Here's how the part is built. I have some questions about the finished solid (model axes, mm). Give positions to 0.01 mm unless a question says otherwise; leave off trailing zeros. Loops run counter-clockwise (first coordinate to the right, second up) from the corner with the lowest first, then second, coordinate; pieces in that order, holes last. Notation, with made-up numbers: (-30, -34.75) - (3, -34.75) arc R31 ccw to (3, -4.75) - close; hole circle Ø3 at (-6.75, 86.25). An arc over 180 degrees is marked (long way). Use one line per item in the form item = value.
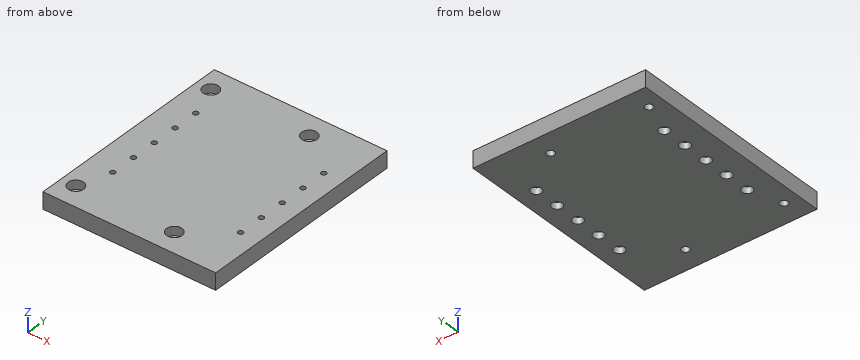
from build123d import *

# Parameters (mm, degrees)
F0_W     = 135
F0_H     = 165
F0_R     = 6
F0_R_2   = 2
F0_R_3   = 3
F1_DEPTH = 13
F2_R     = 6
F3_DEPTH = 7
F4_R     = 4
F5_DEPTH = 5


with BuildPart() as f1:
    # F0 (on Top) → F1 (new body)
    with BuildSketch(Plane.XY):
        with Locations((17.5, 0)):
            Rectangle(F0_W, F0_H)
        with Locations((-38.5, -65)):
            Circle(F0_R, mode=Mode.SUBTRACT)
        with Locations((-30, -40)):
            Circle(F0_R_2, mode=Mode.SUBTRACT)
        with Locations((-30, -20)):
            Circle(F0_R_2, mode=Mode.SUBTRACT)
        with Locations((38.5, -65)):
            Circle(F0_R, mode=Mode.SUBTRACT)
        with Locations((70, -40)):
            Circle(F0_R_2, mode=Mode.SUBTRACT)
        with Locations((70, -20)):
            Circle(F0_R_2, mode=Mode.SUBTRACT)
        with Locations((-30, 0)):
            Circle(F0_R_2, mode=Mode.SUBTRACT)
        with Locations((-30, 20)):
            Circle(F0_R_2, mode=Mode.SUBTRACT)
        with Locations((-30, 40)):
            Circle(F0_R_2, mode=Mode.SUBTRACT)
        with Locations((-38.5, 65)):
            Circle(F0_R, mode=Mode.SUBTRACT)
        with Locations((70, 0)):
            Circle(F0_R_2, mode=Mode.SUBTRACT)
        with Locations((70, 20)):
            Circle(F0_R_2, mode=Mode.SUBTRACT)
        with Locations((70, 40)):
            Circle(F0_R_2, mode=Mode.SUBTRACT)
        with Locations((38.5, 65)):
            Circle(F0_R, mode=Mode.SUBTRACT)
        with Locations((-38.5, 65)):
            Circle(F0_R)
        with Locations((-38.5, 65)):
            Circle(F0_R_3, mode=Mode.SUBTRACT)
        with Locations((38.5, 65)):
            Circle(F0_R)
        with Locations((38.5, 65)):
            Circle(F0_R_3, mode=Mode.SUBTRACT)
        with Locations((38.5, -65)):
            Circle(F0_R)
        with Locations((38.5, -65)):
            Circle(F0_R_3, mode=Mode.SUBTRACT)
        with Locations((-38.5, -65)):
            Circle(F0_R)
        with Locations((-38.5, -65)):
            Circle(F0_R_3, mode=Mode.SUBTRACT)
    extrude(amount=-F1_DEPTH)

    # F0 (on Top) + F2 (on face) → F3 (cut)
    with BuildSketch(Plane.XY):
        with Locations((-38.5, 65)):
            Circle(F0_R)
        with Locations((-38.5, 65)):
            Circle(F0_R_3, mode=Mode.SUBTRACT)
        with Locations((-38.5, 65)):
            Circle(F0_R_3)
        with Locations((38.5, 65)):
            Circle(F0_R)
        with Locations((38.5, 65)):
            Circle(F0_R_3, mode=Mode.SUBTRACT)
        with Locations((38.5, 65)):
            Circle(F0_R_3)
        with Locations((-38.5, -65)):
            Circle(F0_R)
        with Locations((-38.5, -65)):
            Circle(F0_R_3, mode=Mode.SUBTRACT)
        with Locations((38.5, -65)):
            Circle(F0_R)
        with Locations((38.5, -65)):
            Circle(F0_R_3, mode=Mode.SUBTRACT)
        with Locations((38.5, -65)):
            Circle(F0_R_3)
    with BuildSketch(Plane.XY):
        with Locations((-38.5, 65)):
            Circle(F2_R)
        with Locations((-38.5, -65)):
            Circle(F2_R)
    extrude(amount=-F3_DEPTH, mode=Mode.SUBTRACT)

    # F4 (on face) → F5 (cut)
    with BuildSketch(Plane(origin=(0, 0, -13), x_dir=(1, 0, 0), z_dir=(0, 0, -1))):
        with Locations((-30, 40)):
            Circle(F4_R)
        with Locations((-30, 20)):
            Circle(F4_R)
        with Locations((-30, 0)):
            Circle(F4_R)
        with Locations((-30, -20)):
            Circle(F4_R)
        with Locations((-30, -40)):
            Circle(F4_R)
        with Locations((70, 40)):
            Circle(F4_R)
        with Locations((70, 0)):
            Circle(F4_R)
        with Locations((70, -20)):
            Circle(F4_R)
        with Locations((70, -40)):
            Circle(F4_R)
        with Locations((70, 20)):
            Circle(F4_R)
    extrude(amount=-F5_DEPTH, mode=Mode.SUBTRACT)


solid = f1.part
(1) If we section it at A-A (z = -11): Give the number of separate pieces and of enclosed holes in the cut face, plus the area to 3 significant figures.
Geometry says:
separate_pieces = 1
enclosed_holes = 14
area = 21,700 mm²
(2) If I drill on probe 1 along X at (y, z) = (-20, -9.65); probe 2 along Y at (x, z) = (70, -2.5); probe 3 along Y at (x, z) = (-30, -11.9), over which ranges is the centre line in solid material (lowest first)?
Geometry says:
probe_1 = -50 to -34, -26 to 66, 74 to 85
probe_2 = -82.5 to -42, -38 to -22, -18 to -2, 2 to 18, 22 to 38, 42 to 82.5
probe_3 = -82.5 to -44, -36 to -24, -16 to -4, 4 to 16, 24 to 36, 44 to 82.5
(3) If we section it at C-C (y = 40): List the corners of the cut face in (x, z) for me, plus the area to 3 significant figures.
Geometry says:
outline = (-50, -13) - (-34, -13) - (-34, -8) - (-32, -8) - (-32, 0) - (-50, 0) - close; (-28, -8) - (-26, -8) - (-26, -13) - (66, -13) - (66, -8) - (68, -8) - (68, 0) - (-28, 0) - close; (72, -8) - (74, -8) - (74, -13) - (85, -13) - (85, 0) - (72, 0) - close
area = 1,610 mm²
(4) If we section it at B-B (x = 38.5): List the corners of the cut face in (y, z) for me, plus the area to 4 significant figures.
Geometry says:
outline = (-82.5, -13) - (-68, -13) - (-68, -7) - (-71, -7) - (-71, 0) - (-82.5, 0) - close; (-62, -13) - (62, -13) - (62, -7) - (59, -7) - (59, 0) - (-59, 0) - (-59, -7) - (-62, -7) - close; (68, -13) - (82.5, -13) - (82.5, 0) - (71, 0) - (71, -7) - (68, -7) - close
area = 1,905 mm²
(5) For P1, Ø5, axis at x = -30, y = -20, coming from the -Z side, with a flat end and sliding along its axis, tell me the tip position at first contact or that it passes through.
Geometry says:
P1 = -8
